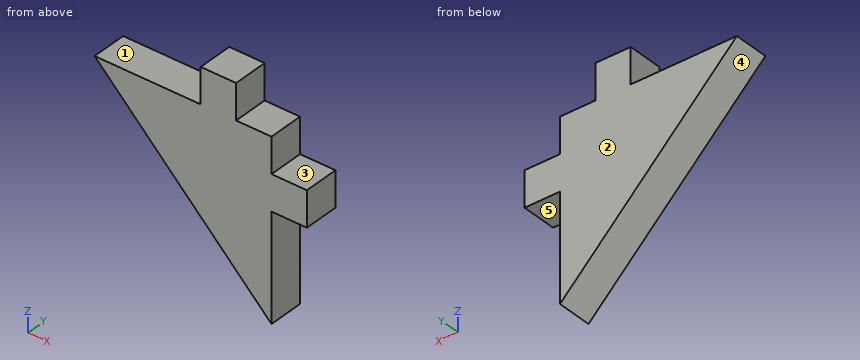
```python
from build123d import *

# Parameters (mm, degrees)
BOSS_EXTRUDE1_DEPTH = 2.54
SKETCH2_W           = 2.54
SKETCH2_H           = 2.54
BOSS_EXTRUDE2_DEPTH = 2.54


with BuildPart() as part:
    # Sketch1 → Boss-Extrude1 (new body)
    with BuildSketch(Plane(origin=(0, 0, 0), x_dir=(1, 0, 0), z_dir=(0, 1, 0))):
        Polygon((0, 0), (0, 12.7), (-12.7, 0), align=None)
    extrude(amount=BOSS_EXTRUDE1_DEPTH)

    # Sketch2 → Boss-Extrude2 (add)
    with BuildSketch(Plane(origin=(0, 2.54, 0), x_dir=(1, 0, 0), z_dir=(0, 1, 0))):
        with Locations((-3.81, -1.27)):
            Rectangle(SKETCH2_W, SKETCH2_H)
        with Locations((1.27, 3.81)):
            Rectangle(SKETCH2_W, SKETCH2_H)
    extrude(amount=-BOSS_EXTRUDE2_DEPTH)


solid = part.part
```
The listing builds one solid part. Answer for the finished solid, in the listing's coordinates (mm). Face numbers are marked on the shaded views. A direction names the side the tool comes from. Round coordinates to 2 decimals unless told otherwise and drop trailing zeros. Order: outer loops, then holes, each group sorted by start corner. A loop starts at its lowest first (then second) coordinate and runs counter-clockwise, first axis right, second up. Notation, with made-up numbers: (14, 86) -> (45, 86) arc R20 ccw to (45, 116) -> close; hole circle Ø11 at (14.25, -36). An arc over 180 degrees is marked (long way). Answer as CSV lines item,"result". Start each with the question number.
(1) Find the intervals of material crossed by probe 1 along X at (y, z) = (2.35, 1.5); probe 2 along Z at (x, y) = (-4.5, 2.2), in increasing order. Write a range as from..to.
(2) The part is cut by section A-A (y = 0.25). Determine the outline of the cut face in (x, z), then the cut area to 3 significant figures.
(3) A tool of negligible diameter and unlimited length cuts with its end or side. For the marked faces 1, 2, 3, 4 and 5, from which of +Z, -Z, +X, -X, +Y, -Y can it reach the whole face along a straight path? Write none if from no direction.
(4) The part is cut by section B-B (x = -10.5). Determine the outline of the cut face in (y, z), then the cut area to 3 significant figures.
(5) The part is cut by section C-C (z = -6.5). Determine the outline of the cut face in (x, y), then the cut area to 3 significant figures.
(6) Flat-ended cylindrical pins translate along their axes: pin 1 Ø1 at (x, y) = (-10, 1.5) entering from -Z; pin 2 Ø0.8 at (x, y) = (-1, 1) entering from +Z; pin 3 Ø0.8 at (y, z) = (1.5, 1) entering from -X. Find the tip coordinate at first contact, or state that the pin passes through.
Evaluation:
1,probe 1,"-5.08..-2.54"
1,probe 2,"-8.2..2.54"
2,outline,"(-12.7, 0) -> (0, -12.7) -> (0, -5.08) -> (2.54, -5.08) -> (2.54, -2.54) -> (0, -2.54) -> (0, 0) -> (-2.54, 0) -> (-2.54, 2.54) -> (-5.08, 2.54) -> (-5.08, 0) -> close"
2,area,"93.5 mm²"
3,face 1,"+Z, -X, +Y, -Y"
3,face 2,"+Z, -Z, +X, -X, +Y"
3,face 3,"+Z, +X, +Y, -Y"
3,face 4,"-Z, -X, +Y, -Y"
3,face 5,"-Z, +X, +Y, -Y"
4,outline,"(0, -2.2) -> (2.54, -2.2) -> (2.54, 0) -> (0, 0) -> close"
4,area,"5.59 mm²"
5,outline,"(-6.2, 0) -> (0, 0) -> (0, 2.54) -> (-6.2, 2.54) -> close"
5,area,"15.7 mm²"
6,pin 1,"z = -3.2"
6,pin 2,"z = 0"
6,pin 3,"x = -5.08"
